Geometry: final body of the model. Coordinates: model frame, mm. Give positions to 0.01 mm unless a question says otherwise; leave off trailing zeros. Write each loop counter-clockwise with the first axis right and the second up, starting at its lowest first coordinate (ties: lowest second). Pieces come first, ordered by that corner, then holes. Notation, with made-up numbers: (-3.5, -20) -> (13.5, -20) arc R14 cw to (13.5, -5) -> close; hole circle Ø1 at (69, 56.25). An arc over 180 degrees is marked (long way). Answer as a JSON object with one key per item and string values.
from build123d import *

# Parameters (mm, degrees)
SKETCH_1_R      = 2
EXTRUDE_1_DEPTH = 5


with BuildPart() as part:
    # 草图1 → 凸台-拉伸1 (new body)
    with BuildSketch(Plane(origin=(0, 0, 0), x_dir=(1, 0, 0), z_dir=(0, 1, 0))):
        with BuildLine():
            ThreePointArc((2.008349917, -19.728571429), (0, -20.5), (-2.008349917, -19.728571429))
            Line((-2.008349917, -19.728571429), (-10.711199556, -11.885714286))
            ThreePointArc((-10.711199556, -11.885714286), (-16, 0), (-10.711199556, 11.885714286))
            Line((-10.711199556, 11.885714286), (-2.008349917, 19.728571429))
            ThreePointArc((-2.008349917, 19.728571429), (0, 20.5), (2.008349917, 19.728571429))
            Line((2.008349917, 19.728571429), (10.711199556, 11.885714286))
            ThreePointArc((10.711199556, 11.885714286), (16, 0), (10.711199556, -11.885714286))
            Line((10.711199556, -11.885714286), (2.008349917, -19.728571429))
        make_face()
        with Locations(Location((0, 17.5, 0), (0, 0, 270))):
            Circle(SKETCH_1_R, mode=Mode.SUBTRACT)
        with Locations(Location((0, -17.5, 0), (0, 0, 270))):
            Circle(SKETCH_1_R, mode=Mode.SUBTRACT)
    extrude(amount=EXTRUDE_1_DEPTH)


solid = part.part
Q1. Material intervals for L1, parallel to X at y = 1.75, z = -17.5; L2, parallel to Z at x = 13.5, y = 1.7; L3, parallel to Z at x = 11.5, y = 2.5, sorted ascending. Write a range as from..to.
Values:
{"L1": "-4.48..-2, 2..4.48", "L2": "-8.59..8.59", "L3": "-11.12..11.12"}
Q2. Mould query, pull axis X, two halves, no side actions, for faces 1 (the cylindrical face through (-16, 2, 0)), 2 (the flat face through (6.3, 2.46, -15.86)), 3 (the cylindrical face through (-1.2, 2.5, 15.9)). Classes: pulls with the +X half, pulls with the -X half, needs draft (parallel to the pull), parting line crosses it, or undercut.
Values:
{"face 1": "pulls with the -X half", "face 2": "pulls with the +X half", "face 3": "undercut"}
Q3. First-contact query: P1, Ø2, axis at x = 7, y = 1.5, coming from the -Z side; P2, Ø8, axis at x = -1.5, z = 5.5, coming from the -Y side; P3, Ø1.5, axis at y = 1, z = -11, coming from the -X side. Flat tips, straight axial feed; report the tip coordinate or a pass-through.
Values:
{"P1": "z = -16.13", "P2": "y = 0", "P3": "x = -12.29"}
Q4. Cut plane D-D (x = -6.5). Return the cut outline in (y, z), and give its area (3 significant figures).
Values:
{"outline": "(0, -15.68) -> (5, -15.68) -> (5, 15.68) -> (0, 15.68) -> close", "area": "157 mm²"}
Q5. Cut plane C-C (y = 3). Return the cut outline in (x, z).
Values:
{"outline": "(-10.71, -11.89) -> (-2.01, -19.73) arc R3 ccw to (2.01, -19.73) -> (10.71, -11.89) arc R16 ccw to (10.71, 11.89) -> (2.01, 19.73) arc R3 ccw to (-2.01, 19.73) -> (-10.71, 11.89) arc R16 ccw to start; hole circle Ø4 at (0, -17.5); hole circle Ø4 at (0, 17.5)"}
Q6. Cut plane A-A (x = 0). Return the cut outline in (y, z), and give its area (3 significant figures).
Values:
{"outline": "(0, -20.5) -> (5, -20.5) -> (5, -19.5) -> (0, -19.5) -> close; (0, -15.5) -> (5, -15.5) -> (5, 15.5) -> (0, 15.5) -> close; (0, 19.5) -> (5, 19.5) -> (5, 20.5) -> (0, 20.5) -> close", "area": "165 mm²"}
Q7. Cut plane B-B (z = 17.5). Return the cut outline in (x, y), and give its area (3 significant figures).
Values:
{"outline": "(-4.48, 0) -> (-2, 0) -> (-2, 5) -> (-4.48, 5) -> close; (2, 0) -> (4.48, 0) -> (4.48, 5) -> (2, 5) -> close", "area": "24.8 mm²"}
